Model file for the job. Use its own axes, mm. Face numbers are marked on the shaded views. A direction names the side the tool comes from. Give positions to 0.01 mm unless a question says otherwise; leave off trailing zeros. Write each loop counter-clockwise with the first axis right and the second up, starting at its lowest first coordinate (ties: lowest second). Pieces come first, ordered by that corner, then holes. Notation, with made-up numbers: (19.5, 37) - (43.5, 37) arc R15 ccw to (43.5, 55) - close; hole circle Ø3 at (-7.5, 83). An arc over 180 degrees is marked (long way). One line per item, written item: value. Start each with the question number.
(1) Cut at D-D, the plane y = 9. List the corners of the cut face in (x, z), and give its area (3 significant figures).
(2) Cut at A-A, the plane y = 0. State how many separate pieces and enclosed holes the cut face has, and give its area (3 significant figures).
(3) Mould opens along X. For the marked faces 1, 2 and 3 say: pulls with the +X half, pulls with the -X half, needs draft (parallel to the pull), parting line crosses it, or undercut.
(4) Drop flat-ended pins along their axis: P1, Ø4, axis at x = 0, y = 18.5, coming from the -Z side; P2, Ø5, axis at x = -4, z = -4, coming from the +Y side; P3, Ø6, axis at x = 1, z = -1.5, coming from the -Y side. Give the stop position or say it passes through.
(5) Cut at C-C, the plane x = 18. List the corners of the cut face in (y, z).
(6) Probe L1, parallel to Y at x = 0, z = 1.5; L2, parallel to X at y = 0, z = -5.2. List the from-to ranges inside material, lowest first.
(7) 3-axis set-ups, long thin cutter, end or side, ignore diameter. For the marked faces 4 and 5: which of +Z, -Z, +X, -X, +Y, -Y reach the whole face in a straight line?
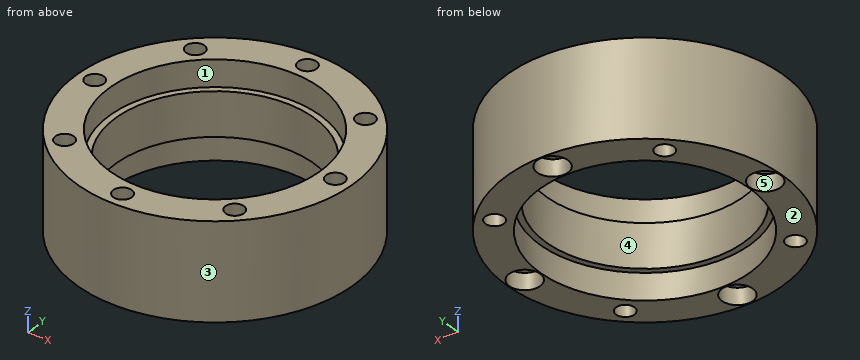
from build123d import *

# Parameters (mm, degrees)
SKETCH3_R          = 1.4
CUT_EXTRUDE2_DEPTH = 8.3
CUT_EXTRUDE4_START = -2.5
SKETCH4_R          = 2.35
CUT_EXTRUDE4_DEPTH = 3.5
CHAMFER1_SIZE      = 0.1
CIRPATTERN3_COUNT  = 4
CIRPATTERN2_COUNT  = 8


with BuildPart() as part:
    # Sketch7 → Revolve1 (revolve)
    with BuildSketch(Plane(origin=(0, 0, 0), x_dir=(1, 0, 0), z_dir=(0, 1, 0))):
        Polygon((16, 7.3), (16, 3.3), (15.07, 3.3), (15.07, -3.3), (16, -3.3), (16, -7.3), (21, -7.3), (21, 7.3), align=None)
    revolve(axis=Axis((0, 0, 8.03), (0, 0, -1)))

    # Sketch3 → Cut-Extrude2 (cut, symmetric)
    with BuildSketch(Plane.XY):
        with Locations((0, 18.5)):
            Circle(SKETCH3_R)
    cut_extrude2 = extrude(amount=CUT_EXTRUDE2_DEPTH, both=True, mode=Mode.SUBTRACT)

    # Sketch4 → Cut-Extrude4 (cut)
    with BuildSketch(Plane(origin=(0, 0, -7.3), x_dir=(-1, 0, 0), z_dir=(0, 0, -1)).offset(CUT_EXTRUDE4_START)):
        with Locations((0, 18.5)):
            Circle(SKETCH4_R)
    cut_extrude4 = extrude(amount=CUT_EXTRUDE4_DEPTH, mode=Mode.SUBTRACT)

    # Chamfer1
    chamfer1_edges = [part.edges().sort_by_distance(p)[0] for p in [
        (-1.4, 18.5, -4.8),
    ]]
    chamfer(chamfer1_edges, length=CHAMFER1_SIZE)

    # CirPattern3: Cut-Extrude4 ×4 about axis
    cirpattern3_axis = Axis((0, 0, 0), (0, 0, 1))
    for i in range(1, CIRPATTERN3_COUNT):
        add(cut_extrude4.rotate(cirpattern3_axis, i * 360 / CIRPATTERN3_COUNT), mode=Mode.SUBTRACT)

    # CirPattern2: Cut-Extrude2 ×8 about axis
    cirpattern2_axis = Axis((0, 0, 0), (0, 0, 1))
    for i in range(1, CIRPATTERN2_COUNT):
        add(cut_extrude2.rotate(cirpattern2_axis, i * 360 / CIRPATTERN2_COUNT), mode=Mode.SUBTRACT)


solid = part.part
Answers follow:
1. outline: (-18.97, -7.3) - (-13.23, -7.3) - (-13.23, -3.3) - (-12.09, -3.3) - (-12.09, 3.3) - (-13.23, 3.3) - (-13.23, 7.3) - (-18.97, 7.3) - close; (12.09, -3.3) - (13.23, -3.3) - (13.23, -7.3) - (18.97, -7.3) - (18.97, 7.3) - (13.23, 7.3) - (13.23, 3.3) - (12.09, 3.3) - close
1. area: 183 mm²
2. separate pieces: 4
2. enclosed holes: 0
2. area: 67.0 mm²
3. face 1: undercut
3. face 2: needs draft
3. face 3: parting line crosses it
4. P1: stops at z = -4.8
4. P2: stops at y = 20.95
4. P3: stops at y = -21
5. outline: (-10.82, -7.3) - (-2.3, -7.3) - (-2.3, -4.8) - (-1.31, -4.8) - (-1.31, 7.3) - (-10.82, 7.3) - close; (1.31, -4.8) - (2.3, -4.8) - (2.3, -7.3) - (10.82, -7.3) - (10.82, 7.3) - (1.31, 7.3) - close
6. L1: y = -21 to -19.9, -17.1 to -15.07, 15.07 to 17.1, 19.9 to 21
6. L2: x = -21 to -20.85, -16.15 to -16, 16 to 16.15, 20.85 to 21
7. face 4: +Z, -Z
7. face 5: -Z
